Part model, mm, in its own coordinate system. A direction names the side the tool comes from. Give positions to 0.01 mm unless a question says otherwise; leave off trailing zeros. Loops run counter-clockwise (first coordinate to the right, second up) from the corner with the lowest first, then second, coordinate; pieces in that order, holes last. Notation, with made-up numbers: M 79.25,1 L 93.25,1 A23 ccw 93.25,23 Z; hole C 67.25,6 d8. An arc over 180 degrees is marked long. Answer in a Markdown table with one row per item.
from build123d import *

# Parameters (mm, degrees)
BOX019_W          = 14
BOX019_H          = 14
BOX019_DEPTH      = 8
BOX020_W          = 14
BOX020_H          = 14
BOX020_DEPTH      = 8
BOX021_W          = 37.5
BOX021_H          = 4
BOX021_DEPTH      = 3
BOX022_W          = 37.5
BOX022_H          = 4
BOX022_DEPTH      = 3
CYLINDER023_R     = 0.7
CYLINDER023_DEPTH = 15
CYLINDER024_R     = 0.7
CYLINDER024_DEPTH = 15
CYLINDER025_R     = 0.7
CYLINDER025_DEPTH = 15
CYLINDER026_R     = 0.7
CYLINDER026_DEPTH = 15
BOX013_W          = 9.5
BOX013_H          = 11
BOX013_DEPTH      = 4
CYLINDER009_R     = 3.5
CYLINDER009_DEPTH = 11.5
BOX007_W          = 30
BOX007_H          = 8
BOX007_DEPTH      = 20
FILLET003_R       = 3.9
CYLINDER008_R     = 1.1
CYLINDER008_DEPTH = 30
CYLINDER007_R     = 1.1
CYLINDER007_DEPTH = 30
CYLINDER006_R     = 1.1
CYLINDER006_DEPTH = 30
CYLINDER005_R     = 1.1
CYLINDER005_DEPTH = 30
CYLINDER004_R     = 0.7
CYLINDER004_DEPTH = 40
CYLINDER003_R     = 0.7
CYLINDER003_DEPTH = 40
CYLINDER002_R     = 0.7
CYLINDER002_DEPTH = 40
CYLINDER001_R     = 1.1
CYLINDER001_DEPTH = 30
CYLINDER_R        = 1.6
CYLINDER_DEPTH    = 20
BOX012_W          = 10
BOX012_H          = 10
BOX012_DEPTH      = 20
FILLET008_R       = 2
BOX003_W          = 10
BOX003_H          = 10
BOX003_DEPTH      = 32
BOX_W             = 83
BOX_H             = 20
BOX_DEPTH         = 12
FILLET_R          = 4
BOX002_W          = 83
BOX002_H          = 40
BOX002_DEPTH      = 40
BOX001_W          = 87
BOX001_H          = 42
BOX001_DEPTH      = 32
FILLET004_R       = 2
FILLET005_R       = 2
BOX005_W          = 10
BOX005_H          = 10
BOX005_DEPTH      = 32
FILLET002_R       = 4
FILLET006_R       = 2
BOX004_W          = 10
BOX004_H          = 10
BOX004_DEPTH      = 32
FILLET001_R       = 4
FILLET007_R       = 2


with BuildPart() as cube016:
    # Box019 → Box019 (new body)
    with BuildSketch(Plane(origin=(-39, 35, 16), x_dir=(1, 0, 0), z_dir=(0, 0, 1))):
        with Locations((7, 7)):
            Rectangle(BOX019_W, BOX019_H)
    extrude(amount=BOX019_DEPTH)


with BuildPart() as cube017:
    # Box020 → Box020 (new body)
    with BuildSketch(Plane(origin=(-20, 35, 16), x_dir=(1, 0, 0), z_dir=(0, 0, 1))):
        with Locations((7, 7)):
            Rectangle(BOX020_W, BOX020_H)
    extrude(amount=BOX020_DEPTH)


with BuildPart() as cube018:
    # Box021 → Box021 (new body)
    with BuildSketch(Plane(origin=(-41.5, 20, 12), x_dir=(1, 0, 0), z_dir=(0, 0, 1))):
        with Locations((18.75, 2)):
            Rectangle(BOX021_W, BOX021_H)
    extrude(amount=BOX021_DEPTH)


with BuildPart() as cube019:
    # Box022 → Box022 (new body)
    with BuildSketch(Plane(origin=(-41.5, 30, 12), x_dir=(1, 0, 0), z_dir=(0, 0, 1))):
        with Locations((18.75, 2)):
            Rectangle(BOX022_W, BOX022_H)
    extrude(amount=BOX022_DEPTH)


with BuildPart() as cylinder023:
    # Cylinder023 → Cylinder023 (new body)
    with BuildSketch(Plane(origin=(-38, 26, 2), x_dir=(1, 0, 0), z_dir=(0, 0, 1))):
        Circle(CYLINDER023_R)
    extrude(amount=CYLINDER023_DEPTH)


with BuildPart() as cylinder024:
    # Cylinder024 → Cylinder024 (new body)
    with BuildSketch(Plane(origin=(-26, 26, 2), x_dir=(1, 0, 0), z_dir=(0, 0, 1))):
        Circle(CYLINDER024_R)
    extrude(amount=CYLINDER024_DEPTH)


with BuildPart() as cylinder025:
    # Cylinder025 → Cylinder025 (new body)
    with BuildSketch(Plane(origin=(-19, 26, 2), x_dir=(1, 0, 0), z_dir=(0, 0, 1))):
        Circle(CYLINDER025_R)
    extrude(amount=CYLINDER025_DEPTH)


with BuildPart() as obj1:
    # Cylinder026 → Cylinder026 (new body)
    with BuildSketch(Plane(origin=(-7, 26, 2), x_dir=(1, 0, 0), z_dir=(0, 0, 1))):
        Circle(CYLINDER026_R)
    extrude(amount=CYLINDER026_DEPTH)

    # Fusion005008: union Cube016, Cube017, Cube018, Cube019, Cylinder023, Cylinder024, Cylinder025
    add(cube016.part)
    add(cube017.part)
    add(cube018.part)
    add(cube019.part)
    add(cylinder023.part)
    add(cylinder024.part)
    add(cylinder025.part)


with BuildPart() as cube011:
    # Box013 → Box013 (new body)
    with BuildSketch(Plane(origin=(32, 9, -1), x_dir=(1, 0, 0), z_dir=(0, 0, 1))):
        with Locations((4.75, 5.5)):
            Rectangle(BOX013_W, BOX013_H)
    extrude(amount=BOX013_DEPTH)


with BuildPart() as obj2:
    # Cylinder009 → Cylinder009 (new body)
    with BuildSketch(Plane(origin=(-55, 10, 17), x_dir=(0, 0, -1), z_dir=(1, 0, 0))):
        Circle(CYLINDER009_R)
    extrude(amount=CYLINDER009_DEPTH)


with BuildPart() as fillet003:
    # Box007 → Box007 (new body)
    with BuildSketch(Plane(origin=(20, 26, 14), x_dir=(1, 0, 0), z_dir=(0, 0, 1))):
        with Locations((15, 4)):
            Rectangle(BOX007_W, BOX007_H)
    extrude(amount=BOX007_DEPTH)

    # Fillet003
    fillet003_edges = [fillet003.edges().sort_by_distance(p)[0] for p in [
        (35, 26, 14),
        (35, 34, 14),
    ]]
    fillet(fillet003_edges, radius=FILLET003_R)


with BuildPart() as obj3:
    # Cylinder008 → Cylinder008 (new body)
    with BuildSketch(Plane(origin=(25, 24, 2), x_dir=(1, 0, 0), z_dir=(0, 0, 1))):
        Circle(CYLINDER008_R)
    extrude(amount=CYLINDER008_DEPTH)


with BuildPart() as obj4:
    # Cylinder007 → Cylinder007 (new body)
    with BuildSketch(Plane(origin=(35, 36, 2), x_dir=(1, 0, 0), z_dir=(0, 0, 1))):
        Circle(CYLINDER007_R)
    extrude(amount=CYLINDER007_DEPTH)


with BuildPart() as obj5:
    # Cylinder006 → Cylinder006 (new body)
    with BuildSketch(Plane(origin=(25, 36, 2), x_dir=(1, 0, 0), z_dir=(0, 0, 1))):
        Circle(CYLINDER006_R)
    extrude(amount=CYLINDER006_DEPTH)


with BuildPart() as obj6:
    # Cylinder005 → Cylinder005 (new body)
    with BuildSketch(Plane(origin=(35, 24, 2), x_dir=(1, 0, 0), z_dir=(0, 0, 1))):
        Circle(CYLINDER005_R)
    extrude(amount=CYLINDER005_DEPTH)


with BuildPart() as obj7:
    # Cylinder004 → Cylinder004 (new body)
    with BuildSketch(Plane(origin=(-46.5, 5, 2), x_dir=(1, 0, 0), z_dir=(0, 0, 1))):
        Circle(CYLINDER004_R)
    extrude(amount=CYLINDER004_DEPTH)


with BuildPart() as obj8:
    # Cylinder003 → Cylinder003 (new body)
    with BuildSketch(Plane(origin=(46.5, 5, 2), x_dir=(1, 0, 0), z_dir=(0, 0, 1))):
        Circle(CYLINDER003_R)
    extrude(amount=CYLINDER003_DEPTH)


with BuildPart() as obj9:
    # Cylinder002 → Cylinder002 (new body)
    with BuildSketch(Plane(origin=(2, 37, 2), x_dir=(1, 0, 0), z_dir=(0, 0, 1))):
        Circle(CYLINDER002_R)
    extrude(amount=CYLINDER002_DEPTH)


with BuildPart() as obj10:
    # Cylinder001 → Cylinder001 (new body)
    with BuildSketch(Plane(origin=(36.5, 15, 0), x_dir=(1, 0, 0), z_dir=(0, 0, 1))):
        Circle(CYLINDER001_R)
    extrude(amount=CYLINDER001_DEPTH)


with BuildPart() as obj11:
    # Cylinder → Cylinder (new body)
    with BuildSketch(Plane(origin=(-55, 10, 17), x_dir=(0, 0, -1), z_dir=(1, 0, 0))):
        Circle(CYLINDER_R)
    extrude(amount=CYLINDER_DEPTH)


with BuildPart() as screwholder005:
    # Box012 → Box012 (new body)
    with BuildSketch(Plane(origin=(33, 10, 4), x_dir=(1, 0, 0), z_dir=(0, 0, 1))):
        with Locations((5, 5)):
            Rectangle(BOX012_W, BOX012_H)
    extrude(amount=BOX012_DEPTH)

    # Fillet008
    fillet008_edges = [screwholder005.edges().sort_by_distance(p)[0] for p in [
        (33, 10, 14),
    ]]
    fillet(fillet008_edges, radius=FILLET008_R)


with BuildPart() as cube:
    # Box003 → Box003 (new body)
    with BuildSketch(Plane(origin=(-3, 32, 0), x_dir=(1, 0, 0), z_dir=(0, 0, 1))):
        with Locations((5, 5)):
            Rectangle(BOX003_W, BOX003_H)
    extrude(amount=BOX003_DEPTH)


with BuildPart() as fillet_body:
    # Box → Box (new body)
    with BuildSketch(Plane(origin=(-41.5, 20, 2), x_dir=(1, 0, 0), z_dir=(0, 0, 1))):
        with Locations((41.5, 10)):
            Rectangle(BOX_W, BOX_H)
    extrude(amount=BOX_DEPTH)

    # Fusion: union Cube
    add(cube.part)

    # Fillet
    fillet_edges = [fillet_body.edges().sort_by_distance(p)[0] for p in [
        (-3, 32, 23),
        (7, 32, 23),
    ]]
    fillet(fillet_edges, radius=FILLET_R)


with BuildPart() as boxhollows:
    # Box002 → Box002 (new body)
    with BuildSketch(Plane(origin=(-41.5, 0, 2), x_dir=(1, 0, 0), z_dir=(0, 0, 1))):
        with Locations((41.5, 20)):
            Rectangle(BOX002_W, BOX002_H)
    extrude(amount=BOX002_DEPTH)

    # Cut: cut Fillet body
    add(fillet_body.part, mode=Mode.SUBTRACT)

    # Cut001: cut ScrewHolder005
    add(screwholder005.part, mode=Mode.SUBTRACT)

    # Fusion005009: union obj1, Cube011, obj2, Fillet003, obj3, obj4, obj5, obj6, obj7, obj8, obj9, obj10, obj11
    add(obj1.part)
    add(cube011.part)
    add(obj2.part)
    add(fillet003.part)
    add(obj3.part)
    add(obj4.part)
    add(obj5.part)
    add(obj6.part)
    add(obj7.part)
    add(obj8.part)
    add(obj9.part)
    add(obj10.part)
    add(obj11.part)


with BuildPart() as mainboxcube:
    # Box001 → Box001 (new body)
    with BuildSketch(Plane(origin=(-43.5, 0, 0), x_dir=(1, 0, 0), z_dir=(0, 0, 1))):
        with Locations((43.5, 21)):
            Rectangle(BOX001_W, BOX001_H)
    extrude(amount=BOX001_DEPTH)

    # Fillet004
    fillet004_edges = [mainboxcube.edges().sort_by_distance(p)[0] for p in [
        (-43.5, 42, 16),
        (43.5, 42, 16),
    ]]
    fillet(fillet004_edges, radius=FILLET004_R)

    # Fillet005
    fillet005_edges = [mainboxcube.edges().sort_by_distance(p)[0] for p in [
        (0, 42, 0),
    ]]
    fillet(fillet005_edges, radius=FILLET005_R)


with BuildPart() as screwholder003:
    # Box005 → Box005 (new body)
    with BuildSketch(Plane(origin=(42, 0, 0), x_dir=(1, 0, 0), z_dir=(0, 0, 1))):
        with Locations((5, 5)):
            Rectangle(BOX005_W, BOX005_H)
    extrude(amount=BOX005_DEPTH)

    # Fillet002
    fillet002_edges = [screwholder003.edges().sort_by_distance(p)[0] for p in [
        (52, 0, 16),
        (52, 10, 16),
    ]]
    fillet(fillet002_edges, radius=FILLET002_R)

    # Fillet006
    fillet006_edges = [screwholder003.edges().sort_by_distance(p)[0] for p in [
        (50.828427, 8.828427, 0),
    ]]
    fillet(fillet006_edges, radius=FILLET006_R)


with BuildPart() as pwrbox:
    # Box004 → Box004 (new body)
    with BuildSketch(Plane(origin=(-52, 0, 0), x_dir=(1, 0, 0), z_dir=(0, 0, 1))):
        with Locations((5, 5)):
            Rectangle(BOX004_W, BOX004_H)
    extrude(amount=BOX004_DEPTH)

    # Fillet001
    fillet001_edges = [pwrbox.edges().sort_by_distance(p)[0] for p in [
        (-52, 0, 16),
        (-52, 10, 16),
    ]]
    fillet(fillet001_edges, radius=FILLET001_R)

    # Fillet007
    fillet007_edges = [pwrbox.edges().sort_by_distance(p)[0] for p in [
        (-45, 0, 0),
    ]]
    fillet(fillet007_edges, radius=FILLET007_R)

    # Fusion005003: union MainBoxCube, ScrewHolder003
    add(mainboxcube.part)
    add(screwholder003.part)

    # Cut005: cut BoxHollows
    add(boxhollows.part, mode=Mode.SUBTRACT)


solid = pwrbox.part
(1) Pull direction X, two halves, no side cores. Call faces 5 (the face through (-6, 41, 20)), 6 (the face through (-45.62, 0.6, 0.57)), 7 (the face through (50.859, 8.797, 17.21)), 8 (the face through (-51.4, 4.99, 0.57)): +X half, -X half, draft (parallel to the pull), parting line (faces both ways), or undercut.
Recorded:
| item | result |
|---|---|
| face 5 | undercut |
| face 6 | draft |
| face 7 | +X half |
| face 8 | -X half |
(2) Saw through at A-A (z = 29). Give the number of separate pieces and of enclosed holes in the cut face, plus the area to 3 significant figures.
Recorded:
| item | result |
|---|---|
| separate pieces | 2 |
| enclosed holes | 3 |
| area | 541 mm^2 |
(3) Drill centre lines: line 1 along X through (y, z) = (36, 8); line 2 along X through (y, z) = (39, 20); line 3 along X through (y, z) = (26, 7.75). Where is each one in solid material? Low to high.
Recorded:
| item | result |
|---|---|
| line 1 | x = -43.5 to 23.9, 26.1 to 33.9, 36.1 to 43.5 |
| line 2 | x = -43.5 to -41.5, -3 to 7, 41.5 to 43.5 |
| line 3 | x = -43.5 to -38.7, -37.3 to -26.7, -25.3 to -19.7, -18.3 to -7.7, -6.3 to 43.5 |
(4) Saw through at B-B (y = 15). Write the cut outline in (x, z).
Recorded:
| item | result |
|---|---|
| outline | M -43.5,2 A2 ccw -41.5,0 L 32,0 L 32,2 L -41.5,2 L -41.5,32 L -43.5,32 Z; M 33,4 L 35.4,4 L 35.4,24 L 33,24 Z; M 37.6,4 L 41.5,4 L 41.5,0 A2 ccw 43.5,2 L 43.5,32 L 41.5,32 L 41.5,24 L 37.6,24 Z |
(5) Pin check, flat tips, straight feed: pin 1 Ø4 at (x, y) = (38.5, 12.5) entering from +Z; pin 2 Ø2 at (x, z) = (45, 17) entering from +Y; pin 3 Ø0.6 at (y, z) = (40.5, 21) entering from -X; pin 4 Ø12 at (y, z) = (6.5, 24.5) entering from +X. Stop position of each tip, or through.
Recorded:
| item | result |
|---|---|
| pin 1 | stops at z = 24 |
| pin 2 | stops at y = 10 |
| pin 3 | stops at x = -43.49 |
| pin 4 | stops at x = 52 |
(6) Saw through at C-C (x = -28). Write the cut outline in (y, z), plus the area to 3 significant figures.
Recorded:
| item | result |
|---|---|
| outline | M 0,0 L 40,0 A2 ccw 42,2 L 42,16 L 40,16 L 40,14 L 34,14 L 34,12 L 30,12 L 30,14 L 24,14 L 24,12 L 20,12 L 20,2 L 0,2 Z; M 40,24 L 42,24 L 42,32 L 40,32 Z |
| area | 351 mm^2 |
(7) Which spindle directions (+Z, -Z, +X, -X, +Y, -Y) get a long thin tool onto all of the face, cutting with end or side? Do faces 1 (the face through (-3, 38, 23)), 2 (the face through (46, 10, 17)), 3 (the face through (-23, 32, 12)), 4 (the face through (45.71, 0.6, 0.57)). Say none if no direction does.
Recorded:
| item | result |
|---|---|
| face 1 | +Z, -Y |
| face 2 | +Z, -Z, +X, +Y |
| face 3 | +Z |
| face 4 | -Z, +X, -Y |
